Here's how the part is built. I have some questions about the finished solid (model axes, mm). Face numbers are marked on the shaded views. A direction names the side the tool comes from. Round coordinates to 2 decimals unless told otherwise and drop trailing zeros. Write each loop counter-clockwise with the first axis right and the second up, starting at its lowest first coordinate (ties: lowest second). Pieces come first, ordered by that corner, then holes. Notation, with made-up numbers: (-16, 24) - (15, 24) arc R5 ccw to (15, 33) - close; hole circle Ø8 at (37.5, 12). An arc over 180 degrees is marked (long way). One line per question, with ' | ' between items. Start each with the question number.
(1) Imagine slicing it at B-B (x = 14.5). Write out the boundary of the cut face in (y, z), plus the area to 3 significant figures.
(2) Imagine slicing it at C-C (z = -5). Write out the boundary of the cut face in (x, y), plus the area to 3 significant figures.
(3) For the marked faces 1, 2, 3 and 4, which set-ups out of +Z, -Z, +X, -X, +Y, -Y let a thin tool reach every point of the face, with its end or its side?
(4) Imagine slicing it at A-A (y = 6). Write out the boundary of the cut face in (x, z), plus the area to 3 significant figures.
(5) Imagine slicing it at D-D (y = 0). Write out the boundary of the cut face in (x, z).
(6) If I drill on L1, parallel to Y at x = 19, z = -5; L2, parallel to Z at x = 15.5, y = 0; L3, parallel to Z at x = 21.25, y = 4.75, over which ranges is the centre line in solid material (lowest first)?
(7) Thinking about a two-plate mould opening in Z: for the marked faces 5, 6 and 7, which applies, pulls with the +Z half, pulls with the -Z half, needs draft (parallel to the pull), parting line crosses it, or undercut?
(8) Will these pins go through, and if not, where does the flat tip stop? pin 1 (1.5 mm diameter, centred on y = 4, z = -5, fed in from -X); pin 2 (4 mm diameter, centred on x = 13, z = -5, fed in from +Y).
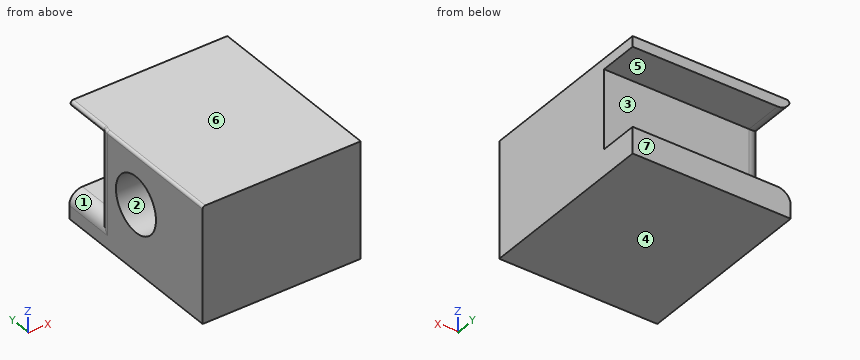
Autodesk Inventor part; units mm, degrees
ref_plane "YZ Plane" through (0, 0, 0) normal (1, 0, 0) x (0, 1, 0)
ref_plane "XZ Plane" through (0, 0, 0) normal (0, 1, 0) x (-1, 0, 0)
ref_plane "XY Plane" through (0, 0, 0) normal (0, 0, 1) x (1, 0, 0)
sketch "Эскиз1" plane through (0, 0, 0) normal (0, 0, 1) x (1, 0, 0)
  line L0 (-0.9994, -4.532) -> (-0.9994, -7)
  line L1 (-0.9994, -7) -> (4.0006, -7)
  line L2 (4.0006, -7) -> (4.0006, 7)
  line L3 (4.0006, 7) -> (1.6539, 7)
  arc A0 (1.6539, 7) -> (-1.5392, 5.8477) centre (1.6539, 2) ccw
  spline S0 degree 3 poles (-1.5392, 5.8477) (-1.841, 5.5961) (-2.3851, 5.1007) (-2.9171, 4.5079) (-3.3417, 3.9411) (-3.598, 3.5113) (-3.8018, 3.0569) (-3.8945, 2.7699) (-3.9568, 2.4926) (-3.9838, 2.3119) (-4.0006, 2.0887) (-4.0006, 1.9113) (-3.9838, 1.6881) (-3.9568, 1.5074) (-3.8945, 1.2301) (-3.8018, 0.9431) (-3.598, 0.4887) (-3.3417, 0.0589) (-2.9342, -0.485) (-2.6405, -0.8158) (-2.428, -1.0328) knots -1 -1 -1 -1 -0.916667 -0.833333 -0.791667 -0.708333 -0.666667 -0.604167 -0.583333 -0.541667 -0.520833 -0.479167 -0.458333 -0.416667 -0.395833 -0.333333 -0.291667 -0.208333 -0.166667 -0.091743 -0.091743 -0.091743 -0.091743
  spline S1 degree 3 poles (-2.428, -1.0328) (-2.2019, -1.2635) (-1.7947, -1.7688) (-1.3413, -2.6303) (-1.0622, -3.563) (-0.9994, -4.209) (-0.9994, -4.532) knots -1 -1 -1 -1 -0.75 -0.5 -0.25 0 0 0 0
  circle A1 centre (28.5006, -1) radius 2.1
  circle A2 centre (-2.1462, 18.5) radius 2.1
  circle A3 centre (-9.0714, -1) radius 2.1
  spline S2 degree 3 poles (-2.4745, 7.8043) (-2.4902, 7.5514) (-2.5538, 7.3036) (-2.7702, 6.8452) (-2.921, 6.6386) (-3.1063, 6.4657) knots 0 0 0 0 0.076038 0.076038 0.152076 0.152076 0.152076 0.152076
  arc A4 (-2.2745, 9.4079) -> (-2.4745, 7.8043) centre (10.5006, 7) ccw
  line L4 (8.0006, -7) -> (40.3538, -7)
  line L5 (40.3538, -7) -> (22.9061, 16.2926)
  arc A5 (22.9061, 16.2926) -> (10.5006, 22.5) centre (10.5006, 7) ccw
  line L6 (10.5006, 22.5) -> (-10.3517, 22.5)
  line L7 (-10.3517, 22.5) -> (-11.2994, 21.5522)
  arc A6 (-11.2994, 21.5522) -> (-11.8548, 20.4853) centre (-9.8852, 20.138) ccw
  line L8 (-11.8548, 20.4853) -> (-11.9558, 19.9127)
  line L9 (-11.9558, 19.9127) -> (-6.1462, 19.9127)
  line L10 (-6.1462, 19.9127) -> (-6.1462, 17.7127)
  line L11 (-6.1462, 17.7127) -> (-12.3437, 17.7127)
  line L12 (-12.3437, 17.7127) -> (-16.3486, -5)
  line L13 (-16.3486, -5) -> (-9.5088, -5)
  line L14 (-9.5088, -5) -> (-9.5088, -7)
  line L15 (-9.5088, -7) -> (-2.4994, -7)
  line L16 (-2.4994, -7) -> (-2.4994, -3.9012)
  spline S3 degree 3 poles (-3.1312, -2.4424) (-2.9413, -2.6206) (-2.7879, -2.8341) (-2.6206, -3.201) (-2.5754, -3.3369) (-2.5147, -3.616) (-2.4994, -3.7584) (-2.4994, -3.9012) knots 0 0 0 0 0.078129 0.078129 0.12097 0.12097 0.16381 0.16381 0.16381 0.16381
  spline S4 degree 2 poles (-3.1312, -2.4424) (-7.8801, 2.0117) (-3.1063, 6.4657) knots -0.944242 -0.944242 -0.944242 -0.053426 -0.053426 -0.053426
  line L17 (23.5006, -7) -> (11.5006, -7)
  line L18 (11.5006, -7) -> (11.5006, 7)
  line L19 (11.5006, 7) -> (23.5006, 7)
  line L20 (23.5006, -7) -> (23.5006, 7)
  spline S5 degree 3 poles (-1.1225, 10.2083) (-1.2509, 10.2303) (-1.3823, 10.2271) (-1.6365, 10.1704) (-1.7568, 10.1175) (-1.9705, 9.9686) (-2.0617, 9.874) (-2.2023, 9.656) (-2.2506, 9.5349) (-2.2745, 9.4079) knots 0 0 0 0 0.039064 0.039064 0.078129 0.078129 0.117193 0.117193 0.155946 0.155946 0.155946 0.155946
  spline S6 degree 2 poles (-1.1225, 10.2083) (8.092, 8.6257) (8.0006, 7) knots 0.047114 0.047114 0.047114 1 1 1
  line L21 (8.0006, 7) -> (8.0006, -7)
  point P0 (0, 0)
  dimension "d0" = 12
extrude "Выдавливание1" add sketch "Эскиз1" against normal blind 10 contours L18 L19 L20 L4
sketch "Эскиз2" plane through (11.5006, -7, 0) normal (-1, 0, 0) x (0, 0, 1)
  line L0 (0, 14) -> (0, 0)
  line L1 (0, 14) -> (-10, 14)
  line L2 (-10, 0) -> (-10, 14)
  line L3 (0, 0) -> (-10, 0)
  line L4 (0, 14) -> (-10, 14)
  line L5 (-5, 14) -> (-5, 0)
  circle A0 centre (-5, 7) radius 2.1
  point P0 (0, 7)
  dimension "d3" = 4.2
extrude "Выдавливание2" cut sketch "Эскиз2" against normal blind 11 contours A0 L5 | L5 A0
sketch "Эскиз3" plane through (11.5006, -7, 0) normal (-1, 0, 0) x (0, 0, 1)
  circle A0 centre (-5, 7) radius 2.1
  line L0 (0, 14) -> (0, 0)
  line L1 (0, 14) -> (-10, 14)
  line L2 (-10, 0) -> (-10, 14)
  line L3 (0, 0) -> (-10, 0)
  line L4 (0, 14) -> (-10, 14)
  line L5 (-2, 14) -> (-8, 14)
  line L6 (-8, 14) -> (-8, 11)
  line L7 (-8, 11) -> (-2, 11)
  line L8 (-2, 11) -> (-2, 14)
  point P0 (0, 7)
  dimension "d6" = 2
  dimension "d7" = 2
  dimension "d8" = 3
extrude "Выдавливание3" cut sketch "Эскиз3" against normal blind 15 contours L8 L7 L6 L1
fillet "Сопряжение1" radius 1 3 edges at (11.5006, 5.5, -8) (11.5006, 4, -5) (11.5006, 5.5, -2)
sketch "Эскиз4" plane through (0, 0, 0) normal (0, 0, 1) x (1, 0, 0)
  line L0 (11.5006, 7) -> (11.5006, -7)
  line L1 (23.5006, 7) -> (11.5006, 7)
  line L2 (23.5006, -7) -> (23.5006, 7)
  line L3 (8.0006, -7) -> (40.3538, -7)
  point P0 (0, 0)
extrude "Выдавливание4" cut sketch "Эскиз4" against normal blind 1.2
fillet "Сопряжение2" radius 0.2 3 edges at (11.5056, 3.1005, -1.2) (11.5006, -2, -1.2) (11.5208, 5.1, -1.2)
properties part number "upor2"
Check sheet entries:
1) outline: (-7, -10) - (7, -10) - (7, -8) - (4, -8) - (4, -2) - (7, -2) - (7, -1.2) - (-7, -1.2) - close; hole circle Ø4.2 at (0, -5) | area: 91.3 mm^2
2) outline: (11.5, -7) - (23.5, -7) - (23.5, 4) - (12.5, 4) arc R1 ccw to (11.5, 3) - (11.5, 2.1) - (22.5, 2.1) - (22.5, -2.1) - (11.5, -2.1) - close | area: 85.6 mm^2
3) face 1: -X, +Y | face 2: -X | face 3: +X, -X, +Y | face 4: -Z, +X, -X, +Y, -Y
4) outline: (11.5, -10) - (23.5, -10) - (23.5, -8) - (12.5, -8) arc R1 ccw to (11.5, -9) - close; (11.63, -1.5) arc R1 ccw to (12.5, -2) - (23.5, -2) - (23.5, -1.2) - (11.81, -1.2) arc R0.2 ccw to start | area: 33.2 mm^2
5) outline: (11.5, -10) - (23.5, -10) - (23.5, -1.2) - (11.7, -1.2) arc R0.2 ccw to (11.5, -1.4) - (11.5, -2.9) - (22.5, -2.9) - (22.5, -7.1) - (11.5, -7.1) - close
6) L1: -7 to -2.1, 2.1 to 4 | L2: -10 to -7.1, -2.9 to -1.2 | L3: -10 to -8, -2 to -1.2
7) face 5: undercut | face 6: pulls with the +Z half | face 7: needs draft
8) pin 1: x = 11.53 | pin 2: y = 4
